Autodesk Inventor part; units mm, degrees
ref_plane "YZ Plane" through (0, 0, 0) normal (1, 0, 0) x (0, 1, 0)
ref_plane "XZ Plane" through (0, 0, 0) normal (0, 1, 0) x (-1, 0, 0)
ref_plane "XY Plane" through (0, 0, 0) normal (0, 0, 1) x (1, 0, 0)
sketch "Szkic1" plane through (0, 0, 0) normal (0, 1, 0) x (-1, 0, 0)
  line L0 (-25.3033, -19.9346) -> (-145.3033, -19.9346)
  line L1 (-145.3033, -19.9346) -> (-145.3033, 80.0654)
  line L2 (-145.3033, 80.0654) -> (14.6967, 80.0654)
  line L3 (14.6967, 80.0654) -> (14.6967, -19.9346)
  line L4 (-25.3033, -19.9346) -> (-25.3033, -59.9346)
  line L5 (14.6967, -59.9346) -> (14.6967, -19.9346)
  line L6 (-1.3707, 111.6296) -> (-1.3707, 118.6296)
  line L7 (-1.3707, 118.6296) -> (-30.3707, 118.6296)
  line L8 (-30.3707, 118.6296) -> (-30.3707, 111.6296)
  line L9 (-1.3707, 111.6296) -> (-30.3707, 111.6296)
  line L10 (14.6967, -59.9346) -> (-25.3033, -59.9346)
  point P0 (0, 0)
  dimension "d0" = 160
  dimension "d1" = 100
  dimension "d2" = 40
  dimension "d3" = 40
  dimension "d9" = 7
  dimension "d39" = 100
extrude "Wyciągnięcie proste1" add sketch "Szkic1" along normal blind 50 contours L0 L1 L2 L3 L5 L10 L4
shell "Skorupa1" thickness 1 removed faces 1 at (51.9699, 50, 46.732)
sketch "Szkic2" plane through (-13.6967, 1, -58.9346) normal (0, 0, 1) x (1, 0, 0)
  line L0 (-1, -1) -> (-1, 49)
  line L1 (39, -1) -> (39, 49)
  line L2 (-1, -1) -> (39, -1)
  line L3 (39, -1) -> (39, 36)
  line L4 (39, 36) -> (4.775, 36)
  line L5 (4.775, 36) -> (39, -1)
  line L6 (-1, -1) -> (39, 36)
  point P0 (13.6967, -1)
  point P1 (19, 17.5)
  dimension "d20" = 37
hole "Otwór1" at (5.3033, 18.5, -58.9346) direction (0, 0, -1) diameter 7 end through all
sketch "Szkic3" plane through (-13.6967, 1, 79.0654) normal (0, 1, 0) x (1, 0, 0)
  line L0 (158, 98) -> (38, 98)
  line L1 (38, 98) -> (0, 98)
  line L2 (0, 0) -> (0, 138)
  line L3 (0, 98) -> (1, 98)
  line L4 (0, 93.0725) -> (8, 93.0725)
  line L5 (8, 93.0725) -> (8, 20.0725)
  line L6 (8, 20.0725) -> (33, 20.0725)
  line L7 (33, 20.0725) -> (33, 93.0725)
  line L8 (33, 93.0725) -> (8, 93.0725)
  line L9 (8, 20.0725) -> (8, 0.0725)
  dimension "d41" = 73
  dimension "d42" = 25
  dimension "d43" = 20
extrude "Wyciągnięcie proste2" cut sketch "Szkic3" against normal blind 10
sketch "Szkic4" plane through (-13.6967, 1, 79.0654) normal (0, 1, 0) x (1, 0, 0)
  line L0 (33, 20.0725) -> (33, 93.0725)
  line L1 (33, 82.5783) -> (33, 67.5783)
  line L2 (33, 67.5783) -> (48, 67.5783)
  line L3 (48, 67.5783) -> (48, 74.5783)
  line L4 (48, 67.5783) -> (55, 67.5783)
  line L5 (55, 67.5783) -> (55, 74.5783)
  line L6 (55, 74.5783) -> (48, 74.5783)
  line L7 (48, 74.5783) -> (48, 67.5783)
  line L8 (55, 67.5783) -> (59, 67.5783)
  line L9 (59, 67.5783) -> (59, 74.5783)
  line L10 (59, 74.5783) -> (66, 74.5783)
  line L11 (66, 74.5783) -> (66, 67.5783)
  line L12 (66, 67.5783) -> (59, 67.5783)
  line L13 (66, 67.5783) -> (70, 67.5783)
  line L14 (70, 67.5783) -> (70, 74.5783)
  line L15 (70, 74.5783) -> (77, 74.5783)
  line L16 (77, 74.5783) -> (77, 67.5783)
  line L17 (77, 67.5783) -> (70, 67.5783)
  point P0 (48, 74.5783)
  dimension "d46" = 15
  dimension "d47" = 15
  dimension "d48" = 7
  dimension "d49" = 7
  dimension "d50" = 4
  dimension "d51" = 7
  dimension "d52" = 4
  dimension "d53" = 7
extrude "Wyciągnięcie proste3" cut sketch "Szkic4" against normal blind 10 contours L3 L6 L5 L4
extrude "Wyciągnięcie proste4" cut sketch "Szkic4" against normal blind 10 contours L14 L15 L16 L17 | L9 L10 L11 L12
properties part number "obudowatuner"
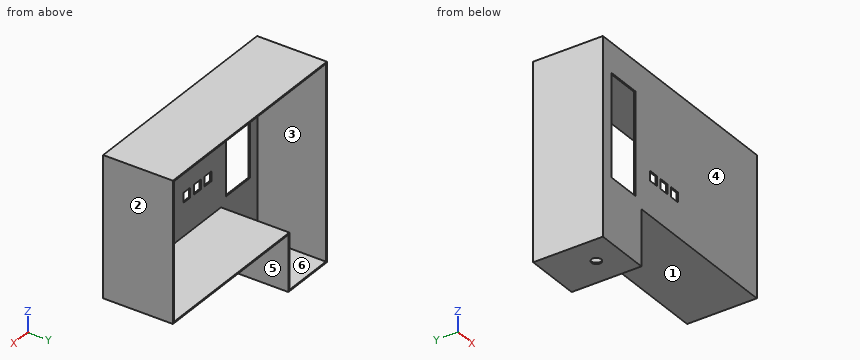
Here's how the part is built. I have some questions about the finished solid (model axes, mm). Face numbers are marked on the shaded views. A direction names the side the tool comes from. Give positions to 0.01 mm unless a question says otherwise; leave off trailing zeros. Write each loop counter-clockwise with the first axis right and the second up, starting at its lowest first coordinate (ties: lowest second). Pieces come first, ordered by that corner, then holes.
(1) Imagine slicing it at C-C, the plane x = 12.5. Write out the boundary of the cut face in (y, z), and give its area (3 significant figures).
Output values:
outline: (0, -59.93) - (50, -59.93) - (50, -58.93) - (1, -58.93) - (1, -14.01) - (0, -14.01) - close; (0, 58.99) - (1, 58.99) - (1, 79.07) - (50, 79.07) - (50, 80.07) - (0, 80.07) - close
area: 165 mm2
(2) If I drill on L1, parallel to X at y = 18.5, z = -59.6; L2, parallel to Z at x = 130, y = 2; L3, parallel to X at y = 15, z = 47, over which ranges is the centre line in solid material (lowest first)?
Output values:
L1: x = -14.7 to 1.8, 8.8 to 25.3
L2: z = -19.93 to -18.93, 79.07 to 80.07
L3: x = -14.7 to -13.7, 144.3 to 145.3
(3) Imagine slicing it at A-A, the plane z = 2.5. Write out the boundary of the cut face in (x, y).
Output values:
outline: (-14.7, 0) - (-5.7, 0) - (-5.7, 1) - (-13.7, 1) - (-13.7, 50) - (-14.7, 50) - close; (19.3, 0) - (145.3, 0) - (145.3, 50) - (144.3, 50) - (144.3, 1) - (19.3, 1) - close
(4) Thinking about a two-plate mould opening in Z: for the marked faces 1, 2 and 3, which applies, pulls with the +Z half, pulls with the -Z half, needs draft (parallel to the pull), parting line crosses it, or undercut?
Output values:
face 1: pulls with the -Z half
face 2: needs draft
face 3: undercut
(5) On a 3-axis mill with a long thin cutter (end or side, diameter ignored), from which of +Z, -Z, +X, -X, +Y, -Y can I reach the whole of each face in a straight line? I mean the marked faces 4, 5 and 6. Say none if no direction works.
Output values:
face 4: +Z, -Z, +X, -X, -Y
face 5: -Z, +X, +Y, -Y
face 6: +Y
(6) Imagine slicing it at D-D, the plane z = 61.5. Write out the boundary of the cut face in (x, y), and give its area (3 significant figures).
Output values:
outline: (-14.7, 0) - (145.3, 0) - (145.3, 50) - (144.3, 50) - (144.3, 1) - (-13.7, 1) - (-13.7, 50) - (-14.7, 50) - close
area: 258 mm2
(7) Imagine slicing it at B-B, the plane y = 40.5. Write out the boundary of the cut face in (x, z).
Output values:
outline: (-14.7, -59.93) - (25.3, -59.93) - (25.3, -19.93) - (145.3, -19.93) - (145.3, 80.07) - (-14.7, 80.07) - close; hole (-13.7, -58.93) - (24.3, -58.93) - (24.3, -18.93) - (144.3, -18.93) - (144.3, 79.07) - (-13.7, 79.07) - close
(8) Will these pins go through, and if not, where does the flat tip stop? pin 1 (4 mm diameter, centred on x = 54, z = -8, fed in from -Y); pin 2 (1.1 mm diameter, centred on x = 47, y = 0.5, fed in from -Z); pin 3 (5 mm diameter, centred on x = 60.5, z = 53.5, fed in from +Y).
Output values:
pin 1: stops at y = 0
pin 2: stops at z = -19.93
pin 3: stops at y = 1
